Here's the drawing with two shaded views (mm, measured from the low corner). I have some questions. A direction names the side the tool comes from. Round coordinates to 2 decimals unless told otherwise and drop trailing zeros. Order: outer loops, then holes, each group sorted by start corner. A loop starts at its lowest first (then second) coordinate and runs counter-clockwise, first axis right, second up.
Q1. If we section it at A-A (y = 6): Please give me the cut outline in (x, z).
Q2. For the marked faces 1 and 2, which set-ups out of +Z, -Z, +X, -X, +Y, -Y let a thin tool reach every point of the face, with its end or its side?
Q3. If we section it at D-D (z = 59): Please give me the cut outline in (x, y).
Q4. Will these pins go through, and if not, where does the flat tip stop? P1, Ø2, axis at x = 8.5, z = 47, coming from the +Y side; P2, Ø2, axis at y = 8.5, z = 55.5, coming from the +X side; P3, Ø3, axis at x = 6, z = 51, coming from the +Y side.
Q5. If we section it at C-C (z = 25.5): Please give me the cut outline in (x, y).
Q6. If I drill on line 1 (Z direction, x = 4.5, y = 1.5); line 2 (Z direction, x = 10.5, y = 2.25); line 3 (Y direction, x = 6.25, z = 73), over which ranges is the centre line in solid material (lowest first)?
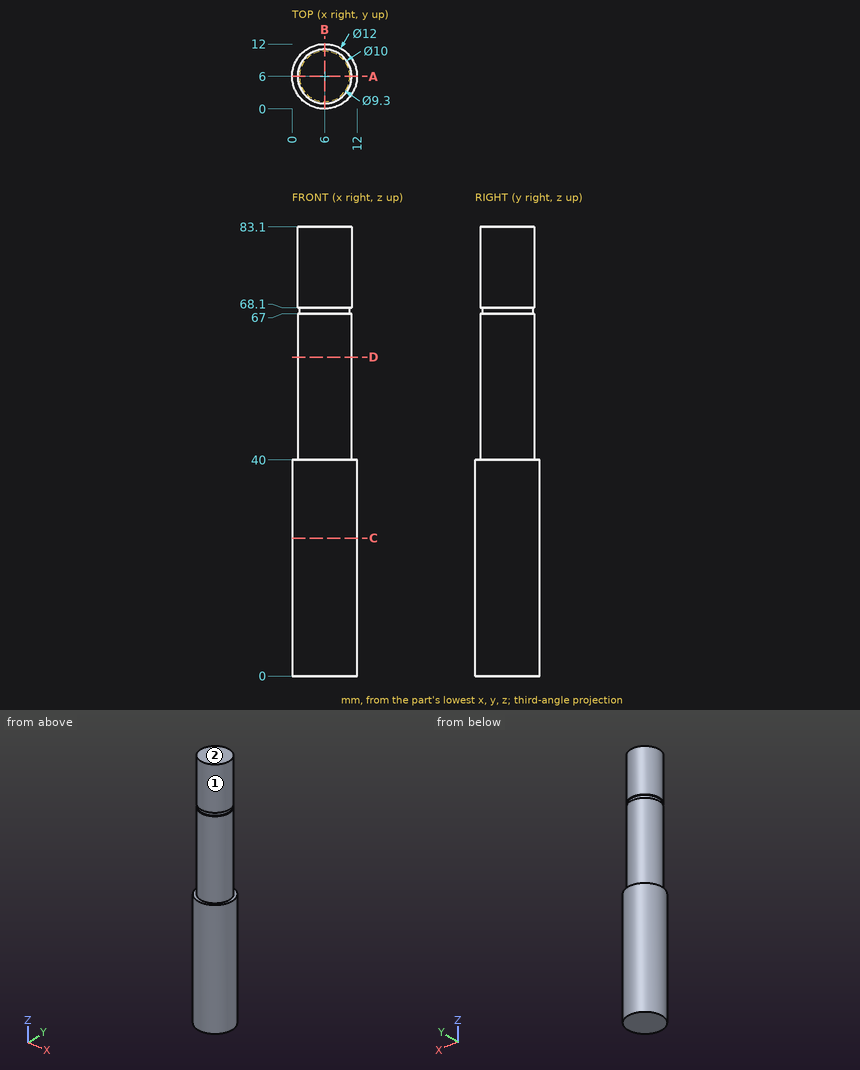
Solution:
1. outline: (0, 0) - (12, 0) - (12, 40) - (11, 40) - (11, 67) - (10.65, 67) - (10.65, 68.1) - (11, 68.1) - (11, 83.1) - (1, 83.1) - (1, 68.1) - (1.35, 68.1) - (1.35, 67) - (1, 67) - (1, 40) - (0, 40) - close
2. face 1: +Z
2. face 2: +Z, +X, -X, +Y, -Y
3. outline: circle Ø10 at (6, 6)
4. P1: stops at y = 10.77
4. P2: stops at x = 10.77
4. P3: stops at y = 11
5. outline: circle Ø12 at (6, 6)
6. line 1: z = 0 to 67, 68.1 to 83.1
6. line 2: z = 0 to 40
6. line 3: y = 1.01 to 10.99
